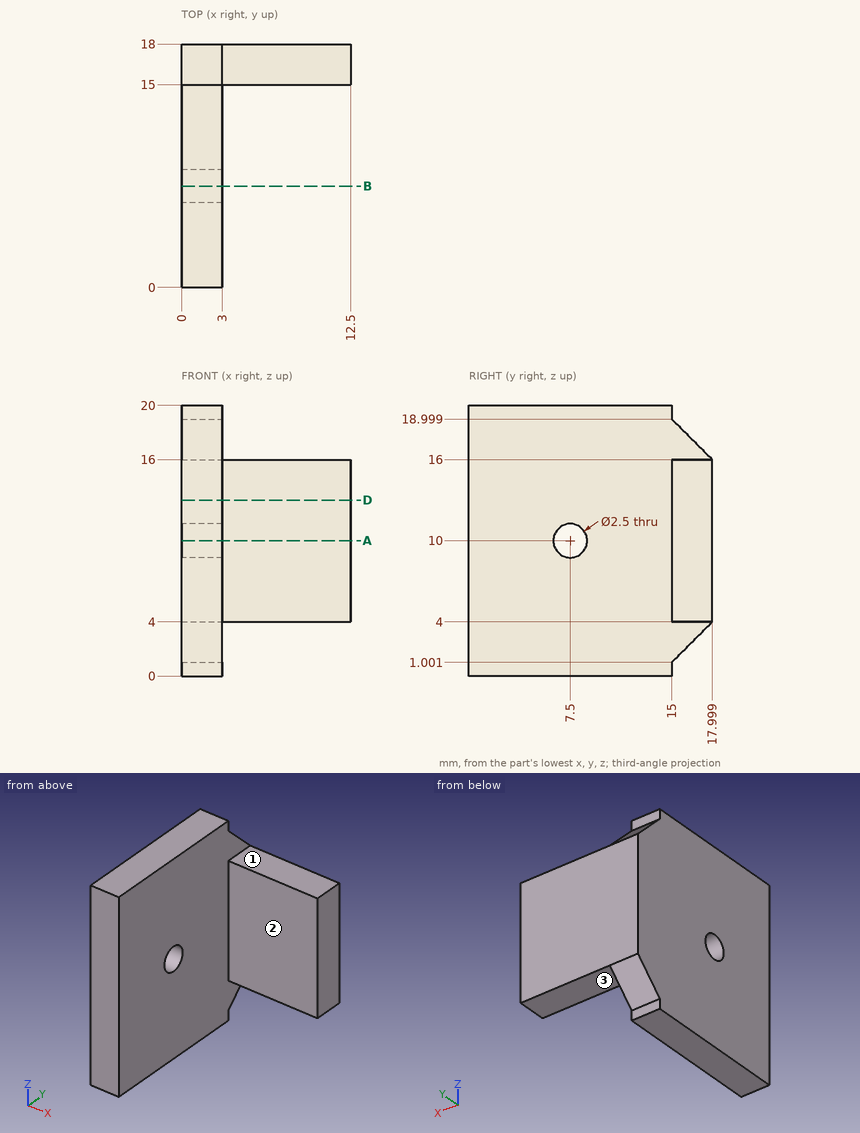
Check sheet for the drawn part. Datum: minimum x, y, z corner. Units: mm. A direction names the side the tool comes from. Give positions to 0.01 mm unless a question says otherwise; leave off trailing zeros. Write each loop counter-clockwise with the first axis right and the second up, starting at its lowest first coordinate (ties: lowest second). Pieces come first, ordered by that corner, then holes. Notation, with made-up numbers: M 47.25,58 L 53.25,58 A23 ccw 53.25,70 Z; hole C 7.5,84.25 d7. An arc over 180 degrees is marked long. Write item = value, one per line.
(1) Access from +Z, -Z, +X, -X, +Y, -Y to the whole of each face (thin tool, end or side, straight path). Record for the marked faces 1, 2 and 3.
Found:
face_1 = +Z, +X, +Y, -Y
face_2 = +Z, -Z, +X, -Y
face_3 = -Z, +X, +Y, -Y
(2) Sectioned sample at A-A (z = 10). Record the cut outline in (x, y).
Found:
outline = M 0,0 L 3,0 L 3,6.25 L 0,6.25 Z; M 0,8.75 L 3,8.75 L 3,15 L 12.5,15 L 12.5,18 L 0,18 Z
(3) Sectioned sample at B-B (y = 7.5). Record the cut outline in (x, z).
Found:
outline = M 0,0 L 3,0 L 3,8.75 L 0,8.75 Z; M 0,11.25 L 3,11.25 L 3,20 L 0,20 Z
(4) Sectioned sample at D-D (z = 13). Record the cut outline in (x, y).
Found:
outline = M 0,0 L 3,0 L 3,15 L 12.5,15 L 12.5,18 L 0,18 Z
(5) Material ranges on line 1 (Z direction, x = 1.6, y = 7.5); line 2 (X direction, y = 13, z = 15); line 3 (Y direction, x = 10.5, z = 13.25), recorded low to high.
Found:
line_1 = 0 to 8.75, 11.25 to 20
line_2 = 0 to 3
line_3 = 15 to 18
(6) Go/stop test with flat-tipped pins: pin 1 Ø6 at (x, z) = (4, 17.5) entering from -Y; pin 2 Ø6 at (x, z) = (11, 12) entering from -Y; pin 3 Ø0.5 at (x, z) = (1, 0.5) entering from +Y; pin 4 Ø9 at (y, z) = (5, 14.5) entering from +X. Record where each tip stops, or that it passes through.
Found:
pin_1 = 0
pin_2 = 15
pin_3 = 15
pin_4 = 3
